The drawing under review shows one solid part. Ordinate dimensions are in mm from its lowest x, y, z. Round coordinates to 2 decimals unless told otherwise and drop trailing zeros. Order: outer loops, then holes, each group sorted by start corner. A loop starts at its lowest first (then second) coordinate and runs counter-clockwise, first axis right, second up.
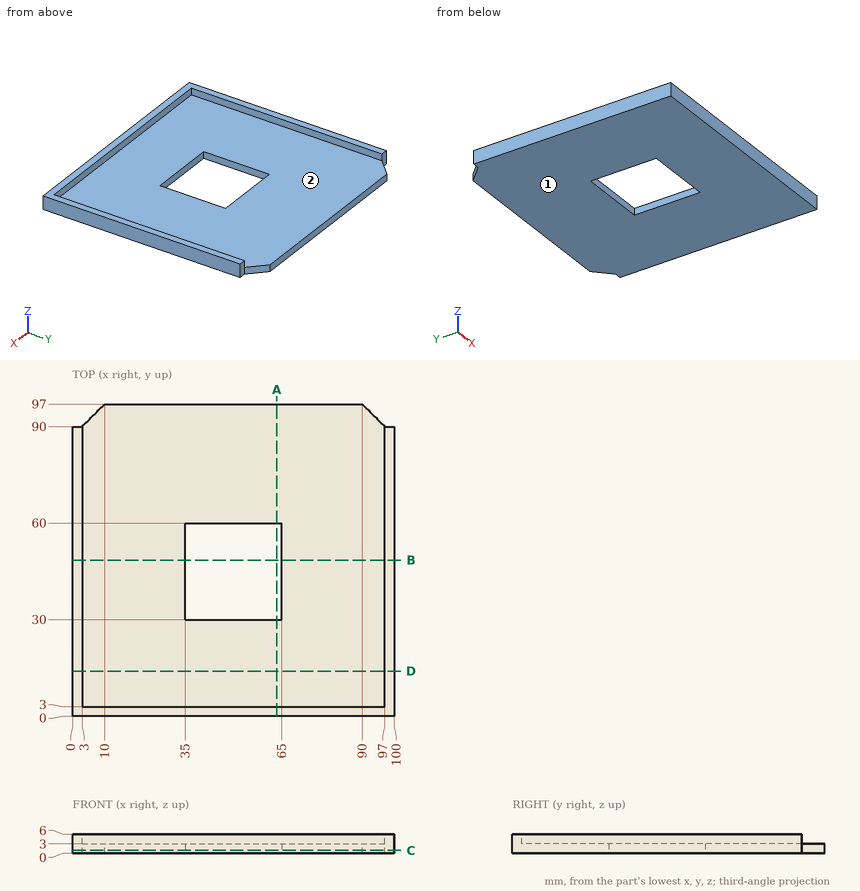
(1) We need section C-C (z = 0.95). Give the boundary of the cut face in (x, y).
(2) We need section B-B (y = 48.5). Give the boundary of the cut face in (x, z).
(3) To check wall thickness, follow L1, parallel to X at y = 16, z = 4.3; L2, parallel to Y at x = 40, z = 1.45; L3, parallel to X at y = 44, z = 2.25. State the ranges of each line that lie inside material, in increasing order.
(4) Clearance check with flat-ended pins moving along their axes: P1, Ø0.9, axis at x = 98, z = 1.5, coming from the +Y side; P2, Ø1, axis at x = 51, z = 5.5, coming from the +Y side; P3, Ø1, axis at x = 65.5, y = 73.5, coming from the +Z side. State where each tip first meets the part, or that it passes through.
(5) We need section D-D (y = 14). Give the boundary of the cut face in (x, z), and give its area (3 significant figures).
(6) The part is to be moulded in two halves that separate along X. For the marked faces 1 and 2, say which applies: pulls with the +X half, pulls with the -X half, needs draft (parallel to the pull), parting line crosses it, or undercut.
(7) We need section A-A (x = 63.5). Give the boundary of the cut face in (y, z), and give its area (3 significant figures).
Verdict:
1. outline: (0, 0) - (100, 0) - (100, 90) - (97, 90) - (90, 97) - (10, 97) - (3, 90) - (0, 90) - close; hole (35, 30) - (65, 30) - (65, 60) - (35, 60) - close
2. outline: (0, 0) - (35, 0) - (35, 3) - (3, 3) - (3, 6) - (0, 6) - close; (65, 0) - (100, 0) - (100, 6) - (97, 6) - (97, 3) - (65, 3) - close
3. L1: x = 0 to 3, 97 to 100
3. L2: y = 0 to 30, 60 to 97
3. L3: x = 0 to 35, 65 to 100
4. P1: stops at y = 90
4. P2: stops at y = 3
4. P3: stops at z = 3
5. outline: (0, 0) - (100, 0) - (100, 6) - (97, 6) - (97, 3) - (3, 3) - (3, 6) - (0, 6) - close
5. area: 318 mm2
6. face 1: needs draft
6. face 2: undercut
7. outline: (0, 0) - (30, 0) - (30, 3) - (3, 3) - (3, 6) - (0, 6) - close; (60, 0) - (97, 0) - (97, 3) - (60, 3) - close
7. area: 210 mm2
